Check sheet for the modelled part. Datum: model origin and axes. Units: mm. Face numbers are marked on the shaded views. A direction names the side the tool comes from. Coordinates: 2 decimals unless noted, no trailing zeros. Write each loop counter-clockwise with the first axis right and the second up, starting at its lowest first coordinate (ties: lowest second). Pieces come first, ordered by that corner, then holes. Notation, with made-up numbers: (5, 45.25) -> (51, 45.25) arc R22 cw to (51, 79.25) -> close; hole circle Ø5 at (45.25, 69). An arc over 180 degrees is marked (long way). Put each result on its own line as item: value.
```python
from build123d import *

# Parameters (mm, degrees)
F0_W      = 121.4898377657
F0_H      = 89.4121006131
F1_DEPTH  = 8.128
F2_R      = 44.6973060351
F3_DEPTH  = 27.686
F4_R      = 31.6381794564
F5_DEPTH  = 71.12
F7_DEPTH  = 12.7
F9_DEPTH  = 15.24
F11_DEPTH = 25.4


with BuildPart() as f1:
    # F0 (on Top) → F1 (new body)
    with BuildSketch(Plane.XY):
        Rectangle(F0_W, F0_H)
    extrude(amount=F1_DEPTH)

    # F2 (on Top) → F3 (join)
    with BuildSketch(Plane.XY):
        with Locations((61.1136257648, 0)):
            Circle(F2_R)
    extrude(amount=F3_DEPTH)

    # F4 (on face) → F5 (cut)
    with BuildSketch(Plane.XY.offset(27.686)):
        with Locations((61.1136257648, 0)):
            Circle(F4_R)
    extrude(amount=-F5_DEPTH, mode=Mode.SUBTRACT)

    # F6 (on face) → F7 (join)
    with BuildSketch(Plane.XY.offset(8.128)):
        with BuildLine():
            Line((17.315906262, -5.9659900144), (17.315906262, 8.9223838266))
            ThreePointArc((17.315906262, 8.9223838266), (16.4414678757, 1.4991585393), (16.8162654603, -5.9659900144))
            Line((16.8162654604, -5.9659900144), (17.315906262, -5.9659900144))
        make_face()
    extrude(amount=F7_DEPTH)

    # F8 (on face) → F9 (join)
    with BuildSketch(Plane.XY.offset(8.128)):
        with BuildLine():
            ThreePointArc((16.9541946333, -6.9133066572), (16.4178062292, 0.3645309758), (17.0728288242, 7.6326516773))
            Line((17.0728288242, 7.6326516773), (-23.0794530362, 7.6326516773))
            Line((-23.0794530362, 7.6326516773), (-23.0794530362, -6.9133066572))
            Line((-23.0794530362, -6.9133066572), (16.9541946333, -6.9133066572))
        make_face()
    extrude(amount=F9_DEPTH)

    # F10 (on face) → F11 (cut)
    with BuildSketch(Plane.XZ.offset(6.9133066572)):
        Polygon((-23.0794530362, 23.368), (-23.0794530362, 8.128), (16.9541946333, 23.368), align=None)
    extrude(amount=-F11_DEPTH, mode=Mode.SUBTRACT)


solid = f1.part
```
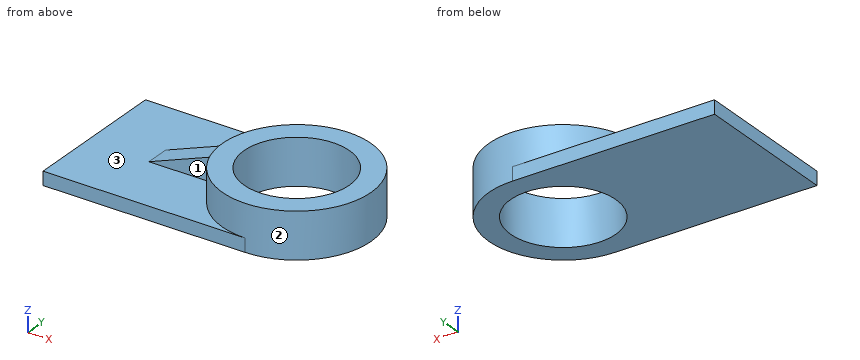
Q1. Material ranges on line 1 along Y through (x, z) = (61.5, 24); line 2 along X through (y, z) = (-17, 24.25); line 3 along X through (y, z) = (-9, 25.75), recorded low to high.
Recorded:
line 1: y = -44.7 to -31.64, 31.64 to 44.7
line 2: x = 19.78 to 34.43, 87.8 to 102.45
line 3: x = 17.33 to 30.78, 91.44 to 104.9
Q2. Cross-section at C-C (x = 89). Record the cut outline in (y, z), plus the area to 3 significant figures.
Recorded:
outline: (-34.93, 0) -> (-14.94, 0) -> (-14.94, 27.69) -> (-34.93, 27.69) -> close; (14.94, 0) -> (34.93, 0) -> (34.93, 27.69) -> (14.94, 27.69) -> close
area: 1,110 mm2
Q3. Tool access check on the marked faces 1, 2 and 3. Record the directions out of +Z, -Z, +X, -X, +Y, -Y that give a thin tool (end or side, any length) a straight path to the whole face; none if there is none.
Recorded:
face 1: +Z, -X, -Y
face 2: +Z
face 3: +Z, -X
Q4. Depth check by flat-ended pin: P1, Ø6, axis at x = 76.5, z = 7.5, coming from the +Y side; P2, Ø10, axis at y = -14, z = 8, coming from the +X side; P3, Ø10, axis at x = 73.5, z = 4.5, coming from the -Y side. Enter the tip coordinate at first touch or a pass-through.
Recorded:
P1: stops at y = 42.95
P2: stops at x = 104.9
P3: stops at y = -44.08
Q5. Cross-section at B-B (y = 0). Record the cut outline in (x, z).
Recorded:
outline: (-60.74, 0) -> (29.48, 0) -> (29.48, 27.69) -> (16.42, 27.69) -> (16.42, 23.37) -> (16.95, 23.37) -> (-23.08, 8.13) -> (-60.74, 8.13) -> close; (92.75, 0) -> (105.81, 0) -> (105.81, 27.69) -> (92.75, 27.69) -> close
Q6. Cross-section at D-D (y = -24.5). Record the cut outline in (x, z), plus the area to 3 significant figures.
Recorded:
outline: (-60.74, 0) -> (41.1, 0) -> (41.1, 27.69) -> (23.73, 27.69) -> (23.73, 8.13) -> (-60.74, 8.13) -> close; (81.13, 0) -> (98.5, 0) -> (98.5, 27.69) -> (81.13, 27.69) -> close
area: 1,650 mm2
